CAD build for the part. Positions are in the model's coordinates, mm. Face numbers are marked on the shaded views. A direction names the side the tool comes from. Give positions to 0.01 mm unless a question says otherwise; leave off trailing zeros. Loops run counter-clockwise (first coordinate to the right, second up) from the corner with the lowest first, then second, coordinate; pieces in that order, holes last.
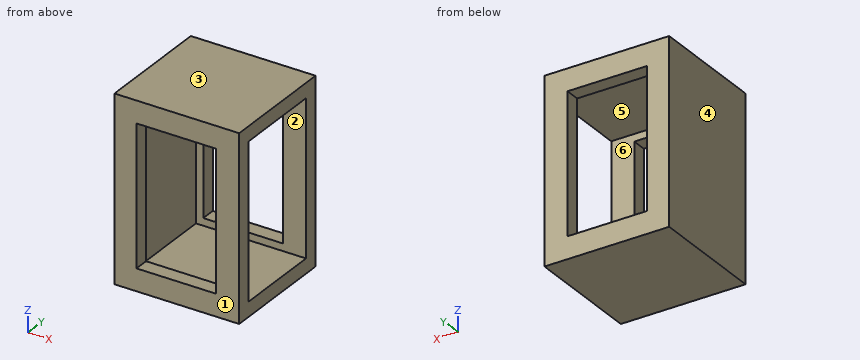
```python
from build123d import *

# Parameters (mm, degrees)
F0_W     = 17
F0_H     = 25
F1_DEPTH = 16
F2_T     = -2
F3_W     = 10.859362
F3_H     = 19
F4_DEPTH = 16.001


with BuildPart() as f1:
    # F0 (on Front) → F1 (new body)
    with BuildSketch(Plane.XZ):
        with Locations((8.5, 12.5)):
            Rectangle(F0_W, F0_H)
    extrude(amount=-F1_DEPTH)

    # F2
    f2_openings = [f1.faces().sort_by_distance(p)[0] for p in [
        (17, 8, 12.5),
    ]]
    offset(amount=F2_T, openings=f2_openings)

    # F3 (on face) → F4 (cut, through all)
    with BuildSketch(Plane(origin=(0, 16, 0), x_dir=(-1, 0, 0), z_dir=(0, 1, 0))):
        with Locations((-8.429681, 12.5)):
            Rectangle(F3_W, F3_H)
    extrude(amount=-F4_DEPTH, mode=Mode.SUBTRACT)


solid = f1.part
```
1. Drop a flat-ended pin along its axis: pin 1 (4 mm diameter, centred on y = 11, z = 17.5, fed in from +X). Give the stop position or say it passes through.
Responses:
pin 1: stops at x = 2
2. Saw through at C-C, the plane x = 15.5. List the corners of the cut face in (y, z).
Responses:
outline: (0, 0) - (16, 0) - (16, 25) - (0, 25) - close; hole (2, 2) - (14, 2) - (14, 23) - (2, 23) - close
3. Pull direction Z, two halves, no side cores. Call the marked faces 3, 4, 5 and 6: released by +Z, released by -Z, zero draft, split by the parting line, or undercut.
Responses:
face 3: released by +Z
face 4: zero draft
face 5: undercut
face 6: undercut
4. Saw through at B-B, the plane x = 4.75. List the corners of the cut face in (y, z), and give its area (3 significant figures).
Responses:
outline: (0, 0) - (16, 0) - (16, 3) - (14, 3) - (14, 2) - (2, 2) - (2, 3) - (0, 3) - close; (0, 22) - (2, 22) - (2, 23) - (14, 23) - (14, 22) - (16, 22) - (16, 25) - (0, 25) - close
area: 72.0 mm2
5. Saw through at D-D, the plane y = 15. List the corners of the cut face in (x, z), and give its area (3 significant figures).
Responses:
outline: (0, 0) - (17, 0) - (17, 25) - (0, 25) - close; hole (3, 3) - (13.86, 3) - (13.86, 22) - (3, 22) - close
area: 219 mm2
6. Probe line 1 along Z through (x, y) = (9.5, 11.5); line 2 along X through (y, z) = (15, 21); line 3 along Z through (x, y) = (7, 1.75). List the from-to ranges inside material, lowest first.
Responses:
line 1: z = 0 to 2, 23 to 25
line 2: x = 0 to 3, 13.86 to 17
line 3: z = 0 to 3, 22 to 25
7. Saw through at A-A, the plane z = 6. List the corners of the cut face in (x, y).
Responses:
outline: (0, 0) - (3, 0) - (3, 2) - (2, 2) - (2, 14) - (3, 14) - (3, 16) - (0, 16) - close; (13.86, 0) - (17, 0) - (17, 2) - (13.86, 2) - close; (13.86, 14) - (17, 14) - (17, 16) - (13.86, 16) - close
8. Tool access for the marked faces 1 and 2: list every direction of +Z, -Z, +X, -X, +Y, -Y with a clear straight run to the whole face (end or side of a thin tool).
Responses:
face 1: +Z, -Z, +X, -X, -Y
face 2: +X
